Source: CAD feature listing. Evaluate the final solid. Frame: model axes, mm. A direction names the side the tool comes from. Round coordinates to 2 decimals unless told otherwise and drop trailing zeros. Write each loop counter-clockwise with the first axis right and the second up, starting at its lowest first coordinate (ties: lowest second). Pieces come first, ordered by that corner, then holes. Notation, with made-up numbers: M 84,30 L 104,30 A17 ccw 104,58 Z; hole C 70.25,-21 d6. An arc over 180 degrees is marked long. Answer in a Markdown table with one row per item. Add a question column.
Item 1: Material intervals for probe 1 along Y at (x, z) = (10, 35); probe 2 along Z at (x, y) = (4.25, 178); probe 3 along Y at (x, z) = (14.25, 48.5), sorted ascending.
Item 2: Set-up query: faces 1 (the face through (5, 226, 87)), 2 (the face through (7.5, 64, 30)), 3 (the face through (11, 212, 88)). Return all of +Z, -Z, +X, -X, +Y, -Y with unobstructed straight access to the full face (end or side cutting, diameter ignored); none if empty.
Item 3: Mould query, pull axis Y, two halves, no side actions, for faces 4 (the face through (7, 0, 96)), 5 (the face through (7, 309, 96)), 6 (the face through (7, 247, 87)), 7 (the face through (0, 152, 99)). Classes: released by +Y, released by -Y, zero draft, split by the parting line, or undercut.
Item 4: Cut plane A-A on y = 221. Return loops of the section in (x, z).
Item 5: Contact query for flat-ended pins moving along their axis: pin 1 (5 mm diameter, centred on y = 178, z = 105, fed in from -X); pin 2 (6.5 mm diameter, centred on y = 193, z = 102.5, fed in from +X). Output: stop coordinate, or through.
Item 6: Cut plane B-B on z = 55.5. Return loops of the section in (x, y), and give its area (3 significant figures).
from build123d import *

# Parameters (mm, degrees)
CROQUIS1_W                 = 309
CROQUIS1_H                 = 195
CROQUIS1_W_2               = 11
CROQUIS1_H_2               = 133
CROQUIS1_W_3               = 9
CROQUIS1_W_4               = 10
SALIENTE_EXTRUIR1_DEPTH    = 15
CROQUIS2_W                 = 67
CROQUIS2_H                 = 133
CORTAR_EXTRUIR2_DEPTH      = 4
CORTAR_EXTRUIR3_DEPTH      = 366.69249377
CORTAR_EXTRUIR3_DEPTH_BACK = 7.5
CROQUIS3_R                 = 2.75


with BuildPart() as part:
    # Croquis1 → Saliente-Extruir1 (new body)
    with BuildSketch(Plane.YZ):
        with Locations((154.5, 97.5)):
            Rectangle(CROQUIS1_W, CROQUIS1_H)
        with Locations((185.5, 87.5)):
            Rectangle(CROQUIS1_W_2, CROQUIS1_H_2, mode=Mode.SUBTRACT)
        with Locations((203.5, 87.5)):
            Rectangle(CROQUIS1_W_3, CROQUIS1_H_2, mode=Mode.SUBTRACT)
        with Locations((221, 87.5)):
            Rectangle(CROQUIS1_W_4, CROQUIS1_H_2, mode=Mode.SUBTRACT)
        with Locations((242, 87.5)):
            Rectangle(CROQUIS1_W_4, CROQUIS1_H_2, mode=Mode.SUBTRACT)
    extrude(amount=SALIENTE_EXTRUIR1_DEPTH)

    # Croquis2 → Cortar-Extruir2 (cut)
    with BuildSketch(Plane.YZ.offset(15)):
        with Locations((213.5, 87.5)):
            Rectangle(CROQUIS2_W, CROQUIS2_H)
    extrude(amount=-CORTAR_EXTRUIR2_DEPTH, mode=Mode.SUBTRACT)

    # Croquis3 → Cortar-Extruir3 (cut, two sides: drawn at the far end of the back side and taken through both)
    with BuildSketch(Plane(origin=(0, 0, 0), x_dir=(0, -1, 0), z_dir=(-1, 0, 0)).offset(-CORTAR_EXTRUIR3_DEPTH_BACK)):
        with Locations(Location((-116, 105, 0), (0, 0, 270))):
            Circle(CROQUIS3_R)
        with Locations(Location((-64, 105, 0), (0, 0, 270))):
            Circle(CROQUIS3_R)
        with Locations(Location((-64, 30, 0), (0, 0, 270))):
            Circle(CROQUIS3_R)
        with Locations((-178, 105)):
            Circle(CROQUIS3_R)
        with Locations((-178, 30)):
            Circle(CROQUIS3_R)
        with Locations(Location((-116, 30, 0), (0, 0, 270))):
            Circle(CROQUIS3_R)
    extrude(amount=CORTAR_EXTRUIR3_DEPTH + CORTAR_EXTRUIR3_DEPTH_BACK, mode=Mode.SUBTRACT)


solid = part.part
Results below:
| question | item | result |
|---|---|---|
| 1 | probe 1 | 0 to 180, 191 to 199, 208 to 216, 226 to 237, 247 to 309 |
| 1 | probe 2 | 0 to 27.25, 32.75 to 102.25, 107.75 to 195 |
| 1 | probe 3 | 0 to 180, 247 to 309 |
| 2 | face 1 | +X, -X |
| 2 | face 2 | -X |
| 2 | face 3 | +X |
| 3 | face 4 | released by -Y |
| 3 | face 5 | released by +Y |
| 3 | face 6 | undercut |
| 3 | face 7 | zero draft |
| 4 | outline | M 0,0 L 15,0 L 15,21 L 0,21 Z; M 0,154 L 15,154 L 15,195 L 0,195 Z |
| 5 | pin 1 | x = 7.5 |
| 5 | pin 2 | x = 11 |
| 6 | outline | M 0,0 L 15,0 L 15,180 L 0,180 Z; M 0,191 L 11,191 L 11,199 L 0,199 Z; M 0,208 L 11,208 L 11,216 L 0,216 Z; M 0,226 L 11,226 L 11,237 L 0,237 Z; M 0,247 L 15,247 L 15,309 L 0,309 Z |
| 6 | area | 3,930 mm2 |
